Geometry: see drawing. Coordinates: mm, zero at the bounding-box minimum. A direction names the side the tool comes from. Give positions to 0.01 mm unless a question says otherwise; leave off trailing zeros. Write each loop counter-clockwise with the first axis right and the second up, starting at its lowest first coordinate (ties: lowest second). Pieces come first, ordered by that corner, then holes. Notation, with made-up numbers: (32, 70) -> (74, 70) arc R15 cw to (74, 94) -> close; hole circle Ø8 at (-39.5, -24). An arc over 180 degrees is marked (long way). Answer as a JSON object with one key per item and string values. Group by question number.
Item 1: Ray query, probe 1 along Y at (x, z) = (28, 25.5); probe 2 along X at (y, z) = (38, 21.5); probe 3 along Y at (x, z) = (23, 26). Return the intervals inside material, ascending. Write a range as from..to.
Item 2: Section query C-C on y = 21. Return the cut outline in (x, z).
Item 3: Section query D-D on z = 9.5. Return the cut outline in (x, y).
Item 4: Section query A-A on z = 27. Return the cut outline in (x, y).
Item 5: Access query for the marked faces 1, 2, 3 and 4. Directions: +Z, -Z, +X, -X, +Y, -Y. A direction counts if a zero-diameter tool reaches every point of the face in a straight line with its end or side. Return the directions, or none.
Item 6: First-contact query: pin 1 Ø2 at (x, z) = (24.5, 10) entering from -Y; pin 2 Ø6 at (y, z) = (30.5, 6) entering from +X; pin 3 Ø12 at (x, y) = (10.5, 25) entering from +Z. Flat tips, straight axial feed; report the tip coordinate or a pass-through.
Item 7: Section query B-B on x = 6. Return the cut outline in (y, z).
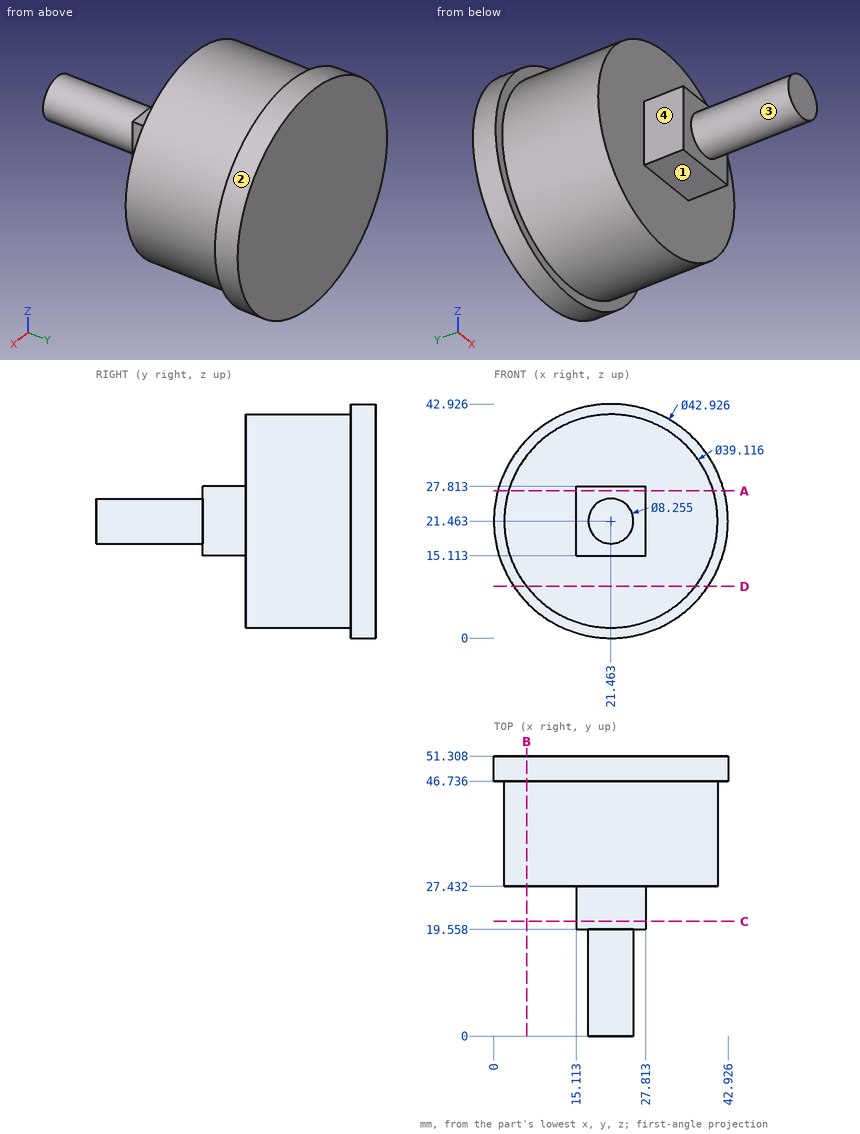
Worked answers:
{
 "1": {"probe 1": "27.43..51.31", "probe 2": "1.91..41.02", "probe 3": "19.56..51.31"},
 "2": {"outline": "(15.11, 15.11) -> (27.81, 15.11) -> (27.81, 27.81) -> (15.11, 27.81) -> close"},
 "3": {"outline": "(3.64, 46.74) -> (5.99, 46.74) -> (5.99, 27.43) -> (36.94, 27.43) -> (36.94, 46.74) -> (39.28, 46.74) -> (39.28, 51.31) -> (3.64, 51.31) -> close"},
 "4": {"outline": "(0.73, 46.74) -> (2.71, 46.74) -> (2.71, 27.43) -> (15.11, 27.43) -> (15.11, 19.56) -> (27.81, 19.56) -> (27.81, 27.43) -> (40.22, 27.43) -> (40.22, 46.74) -> (42.2, 46.74) -> (42.2, 51.31) -> (0.73, 51.31) -> close"},
 "5": {"face 1": "-Z, +X, -X, -Y", "face 2": "+Y, -Y", "face 3": "-Y", "face 4": "+Z, -Z, -X, -Y"},
 "6": {"pin 1": "y = 27.43", "pin 2": "x = 36.54", "pin 3": "z = 40.24"},
 "7": {"outline": "(27.43, 9.49) -> (46.74, 9.49) -> (46.74, 6.58) -> (51.31, 6.58) -> (51.31, 36.35) -> (46.74, 36.35) -> (46.74, 33.44) -> (27.43, 33.44) -> close"}
}
